from build123d import *

# Parameters (mm, degrees)
SKETCH1_W           = 22
SKETCH1_H           = 31
SKETCH1_R           = 1.3
BOSS_EXTRUDE1_DEPTH = 7
SKETCH2_R           = 3.6
CUT_EXTRUDE1_DEPTH  = 10
SKETCH4_W           = 6.98
SKETCH4_H           = 31
CUT_EXTRUDE2_DEPTH  = 4


with BuildPart() as part:
    # Sketch1 → Boss-Extrude1 (new body)
    with BuildSketch(Plane(origin=(0, 0, 0), x_dir=(1, 0, 0), z_dir=(0, 1, 0))):
        Rectangle(SKETCH1_W, SKETCH1_H)
        with Locations((-8, 12.5)):
            Circle(SKETCH1_R, mode=Mode.SUBTRACT)
        with Locations((8, 12.5)):
            Circle(SKETCH1_R, mode=Mode.SUBTRACT)
        with Locations((-8, -12.5)):
            Circle(SKETCH1_R, mode=Mode.SUBTRACT)
        with Locations((8, -12.5)):
            Circle(SKETCH1_R, mode=Mode.SUBTRACT)
    extrude(amount=BOSS_EXTRUDE1_DEPTH)

    # Sketch2 → Cut-Extrude1 (cut)
    with BuildSketch(Plane(origin=(0, 7, 0), x_dir=(1, 0, 0), z_dir=(0, 1, 0))):
        Circle(SKETCH2_R)
    extrude(amount=-CUT_EXTRUDE1_DEPTH, mode=Mode.SUBTRACT)

    # Sketch4 → Cut-Extrude2 (cut)
    with BuildSketch(Plane.XZ):
        with Locations((7.51, 0)):
            Rectangle(SKETCH4_W, SKETCH4_H)
        with Locations((-7.51, 0)):
            Rectangle(SKETCH4_W, SKETCH4_H)
    extrude(amount=-CUT_EXTRUDE2_DEPTH, mode=Mode.SUBTRACT)


solid = part.part
Could you check a few things on this model? Use its own coordinates, in mm. A direction names the side the tool comes from. Give positions to 0.01 mm unless a question says otherwise; leave off trailing zeros. Order: outer loops, then holes, each group sorted by start corner. A loop starts at its lowest first (then second) coordinate and runs counter-clockwise, first axis right, second up. Notation, with made-up numbers: (79, 32) - (87, 32) arc R13 ccw to (87, 53) - close; hole circle Ø1 at (34, 33.5). An arc over 180 degrees is marked (long way). One line per item, written item: value. Start each with the question number.
1. Imagine slicing it at A-A on x = -8.5. List the corners of the cut face in (y, z) for me.
2. Imagine slicing it at B-B on z = 12.5. List the corners of the cut face in (x, y) for me, plus the area to 3 significant figures.
3. Thinking about a two-plate mould opening in Z: for faces 1 (the face through (11, 5, 0)), 2 (the face through (0, 4, -15.5)), 3 (the face through (3.434, 3.549, -1.081)), which applies, +Z half, -Z half, draft (parallel to the pull), parting line (faces both ways), or undercut?
4. For P1, Ø3.5, axis at x = -7.5, z = 6, coming from the -Y side; P2, Ø2, axis at y = 2, z = 2, coming from the -X side; P3, Ø2.5, axis at x = -8, z = -12.5, coming from the +Y side; P4, Ø3, axis at y = 1, z = 5, coming from the +X side, each with a flat end and sliding along its axis, tell me the tip position at first contact or that it passes through.
5. For faces 4 (the face through (4.02, 2, 0)), 5 (the face through (-4.02, 2, 0)), 6 (the face through (0, 7, -4)), which set-ups out of +Z, -Z, +X, -X, +Y, -Y let a thin tool reach every point of the face, with its end or its side?
6. If I drill on probe 1 along Z at (x, y) = (-8, 5); probe 2 along X at (y, z) = (5.65, 12.5); probe 3 along X at (y, z) = (3.75, 0), over which ranges is the centre line in solid material (lowest first)?
7. Imagine slicing it at C-C on x = 0. List the corners of the cut face in (y, z) for me, plus the area to 3 significant figures.
8. Imagine slicing it at D-D on z = 0. List the corners of the cut face in (x, y) for me, plus the area to 3 significant figures.
Values:
1. outline: (4, -15.5) - (7, -15.5) - (7, -13.7) - (4, -13.7) - close; (4, -11.3) - (7, -11.3) - (7, 11.3) - (4, 11.3) - close; (4, 13.7) - (7, 13.7) - (7, 15.5) - (4, 15.5) - close
2. outline: (-11, 4) - (-9.3, 4) - (-9.3, 7) - (-11, 7) - close; (-6.7, 4) - (-4.02, 4) - (-4.02, 0) - (4.02, 0) - (4.02, 4) - (6.7, 4) - (6.7, 7) - (-6.7, 7) - close; (9.3, 4) - (11, 4) - (11, 7) - (9.3, 7) - close
2. area: 82.6 mm²
3. face 1: draft
3. face 2: -Z half
3. face 3: undercut
4. P1: y = 4
4. P2: x = -4.02
4. P3: through
4. P4: x = 4.02
5. face 4: +Z, -Z, +X, -Y
5. face 5: +Z, -Z, -X, -Y
5. face 6: +Z, -Z, +X, -X, +Y
6. probe 1: -15.5 to -13.8, -11.2 to 11.2, 13.8 to 15.5
6. probe 2: -11 to -9.3, -6.7 to 6.7, 9.3 to 11
6. probe 3: -4.02 to -3.6, 3.6 to 4.02
7. outline: (0, -15.5) - (7, -15.5) - (7, -3.6) - (0, -3.6) - close; (0, 3.6) - (7, 3.6) - (7, 15.5) - (0, 15.5) - close
7. area: 167 mm²
8. outline: (-11, 4) - (-4.02, 4) - (-4.02, 0) - (-3.6, 0) - (-3.6, 7) - (-11, 7) - close; (3.6, 0) - (4.02, 0) - (4.02, 4) - (11, 4) - (11, 7) - (3.6, 7) - close
8. area: 47.8 mm²
